from build123d import *

# Parameters (mm, degrees)
SKETCH_1_R      = 32.5
SKETCH_1_R_2    = 6.5
SKETCH_1_R_3    = 1.65
SKETCH_1_R_4    = 1.7
EXTRUDE_1_DEPTH = 3


with BuildPart() as part:
    # 草图1 → 凸台-拉伸1 (new body)
    with BuildSketch(Plane(origin=(0, 0, 0), x_dir=(1, 0, 0), z_dir=(0, 1, 0))):
        with Locations(Location((0, 0, 0), (0, 0, 270))):
            Circle(SKETCH_1_R)
        with Locations(Location((0, 0, 0), (0, 0, 270))):
            Circle(SKETCH_1_R_2, mode=Mode.SUBTRACT)
        with Locations(Location((-7.3, 15.5, 0), (0, 0, 270))):
            Circle(SKETCH_1_R_3, mode=Mode.SUBTRACT)
        with Locations(Location((6.123393759, 7.75, 0), (0, 0, 270))):
            Circle(SKETCH_1_R_3, mode=Mode.SUBTRACT)
        with Locations(Location((6.123393759, -7.75, 0), (0, 0, 270))):
            Circle(SKETCH_1_R_3, mode=Mode.SUBTRACT)
        with Locations(Location((-7.3, -15.5, 0), (0, 0, 270))):
            Circle(SKETCH_1_R_3, mode=Mode.SUBTRACT)
        with Locations(Location((-20.723393759, -7.75, 0), (0, 0, 270))):
            Circle(SKETCH_1_R_3, mode=Mode.SUBTRACT)
        with Locations(Location((-20.723393759, 7.75, 0), (0, 0, 270))):
            Circle(SKETCH_1_R_3, mode=Mode.SUBTRACT)
        with Locations(Location((17.5, 0, 0), (0, 0, 270))):
            Circle(SKETCH_1_R_4, mode=Mode.SUBTRACT)
        with Locations(Location((0, 28, 0), (0, 0, 270))):
            Circle(SKETCH_1_R_3, mode=Mode.SUBTRACT)
        with Locations(Location((24.248711306, 14, 0), (0, 0, 270))):
            Circle(SKETCH_1_R_3, mode=Mode.SUBTRACT)
        with Locations(Location((24.248711306, -14, 0), (0, 0, 270))):
            Circle(SKETCH_1_R_3, mode=Mode.SUBTRACT)
        with Locations(Location((0, -28, 0), (0, 0, 270))):
            Circle(SKETCH_1_R_3, mode=Mode.SUBTRACT)
        with Locations(Location((-24.248711306, -14, 0), (0, 0, 270))):
            Circle(SKETCH_1_R_3, mode=Mode.SUBTRACT)
        with Locations(Location((-24.248711306, 14, 0), (0, 0, 270))):
            Circle(SKETCH_1_R_3, mode=Mode.SUBTRACT)
        with BuildLine():
            ThreePointArc((8.419035512, -20.325349715), (15.556349186, -15.556349186), (20.325349715, -8.419035512))
            ThreePointArc((20.325349715, -8.419035512), (19.242957515, -5.805909582), (16.629831585, -6.888301783))
            ThreePointArc((16.629831585, -6.888301783), (12.727922061, -12.727922061), (6.888301783, -16.629831585))
            ThreePointArc((6.888301783, -16.629831585), (5.805909582, -19.242957515), (8.419035512, -20.325349715))
        make_face(mode=Mode.SUBTRACT)
        with BuildLine():
            ThreePointArc((8.419035512, 20.325349715), (15.556349186, 15.556349186), (20.325349715, 8.419035512))
            ThreePointArc((20.325349715, 8.419035512), (19.242957515, 5.805909582), (16.629831585, 6.888301783))
            ThreePointArc((16.629831585, 6.888301783), (12.727922061, 12.727922061), (6.888301783, 16.629831585))
            ThreePointArc((6.888301783, 16.629831585), (5.805909582, 19.242957515), (8.419035512, 20.325349715))
        make_face(mode=Mode.SUBTRACT)
    extrude(amount=EXTRUDE_1_DEPTH)


solid = part.part
Source: CAD feature listing. Evaluate the final solid. Frame: model axes, mm. Round coordinates to 2 decimals unless told otherwise and drop trailing zeros. Write each loop counter-clockwise with the first axis right and the second up, starting at its lowest first coordinate (ties: lowest second). Pieces come first, ordered by that corner, then holes. Notation, with made-up numbers: (51.25, 58.5) - (76.25, 58.5) arc R12 ccw to (76.25, 69.5) - close; hole circle Ø9 at (67, 37.25). An arc over 180 degrees is marked (long way). Use CSV: the item, a comma, the result in double quotes. Start each with the question number.
(1) Cut plane A-A, the plane x = 0. Return loops of the section in (y, z), and give its area (3 significant figures).
(2) Cut plane D-D, the plane y = 1.05. Give the number of separate pieces and of enclosed holes in the cut face, and give its area (3 significant figures).
(3) Cut plane B-B, the plane z = 0. Return loops of the section in (x, y), and give its area (3 significant figures).
(4) Material intervals for probe 1 along X at (y, z) = (2.25, 0); probe 2 along Z at (x, y) = (23.5, 0.2); probe 3 along X at (y, z) = (2.1, -7.75), sorted ascending. Write a range as [from, to].
(5) First-contact query: pin 1 Ø1 at (x, y) = (-8, 0.5) entering from +Z. Flat tip, straight axial feed; report the tip coordinate or a pass-through.
(6) Mould query, pull axis Z, two halves, no side actions, for faces 1 (the face through (5.79, 1.48, -19.2)), 2 (the face through (9.76, 1.48, 31)), 3 (the face through (0, 0, 7)). Classes: pulls with the +Z half, pulls with the -Z half, needs draft (parallel to the pull), parting line crosses it, or undercut.
(7) Cut plane C-C, the plane x = -7.3. Return loops of the section in (y, z).
Geometry says:
1,outline,"(0, -32.5) - (3, -32.5) - (3, -29.65) - (0, -29.65) - close; (0, -26.35) - (3, -26.35) - (3, -6.5) - (0, -6.5) - close; (0, 6.5) - (3, 6.5) - (3, 26.35) - (0, 26.35) - close; (0, 29.65) - (3, 29.65) - (3, 32.5) - (0, 32.5) - close"
1,area,"136 mm²"
2,separate pieces,"1"
2,enclosed holes,"16"
2,area,"2,920 mm²"
3,outline,"(-32.5, 0) - (-6.5, 0) - (-6.5, 3) - (-32.5, 3) - close; (6.5, 0) - (15.8, 0) - (15.8, 3) - (6.5, 3) - close; (19.2, 0) - (32.5, 0) - (32.5, 3) - (19.2, 3) - close"
3,area,"146 mm²"
4,probe 1,"[-32.5, -6.5], [6.5, 15.8], [19.2, 32.5]"
4,probe 2,"[-22.45, -15.47], [-12.53, 12.53], [15.47, 22.45]"
4,probe 3,"[-31.56, -22.37], [-19.07, 4.47], [7.77, 16.25], [20.48, 31.56]"
5,pin 1,"z = 31.62"
6,face 1,"undercut"
6,face 2,"parting line crosses it"
6,face 3,"needs draft"
7,outline,"(0, -31.67) - (3, -31.67) - (3, -17.15) - (0, -17.15) - close; (0, -13.85) - (3, -13.85) - (3, 13.85) - (0, 13.85) - close; (0, 17.15) - (3, 17.15) - (3, 31.67) - (0, 31.67) - close"
